```python
from build123d import *

# Parameters (mm, degrees)
MODEL_R             = 1.5
BOSS_EXTRUDE1_DEPTH = 3


with BuildPart() as part:
    # Model → Boss-Extrude1 (new body)
    with BuildSketch(Plane.XY):
        with BuildLine():
            Line((0.88624, 25.209039561), (0.88624, 11.208991882))
            ThreePointArc((0.88624, 11.208991882), (13.486238839, -1.391009279), (26.08624, 11.20898956))
            Line((26.08624, 11.20898956), (26.08624, 25.209041884))
            ThreePointArc((26.08624, 25.209041884), (13.486238839, 37.809039561), (0.88624, 25.209039561))
        make_face()
        with Locations((4.586289997, 18.209039557)):
            Circle(MODEL_R, mode=Mode.SUBTRACT)
        with Locations((22.586289997, 18.209039557)):
            Circle(MODEL_R, mode=Mode.SUBTRACT)
        Polygon((19.586238839, 6.708989561), (19.586238839, 29.708989561), (15.886238839, 29.708989561), (15.886238839, 31.708989561), (10.886238839, 31.708989561), (10.886238839, 29.708989561), (7.386238839, 29.708989561), (7.386238839, 6.708989561), align=None, mode=Mode.SUBTRACT)
    extrude(amount=BOSS_EXTRUDE1_DEPTH)


solid = part.part
```
Source: CAD feature listing. Evaluate the final solid. Frame: model axes, mm. A direction names the side the tool comes from. Round coordinates to 2 decimals unless told otherwise and drop trailing zeros. Write each loop counter-clockwise with the first axis right and the second up, starting at its lowest first coordinate (ties: lowest second). Pieces come first, ordered by that corner, then holes. Notation, with made-up numbers: M 34.25,32 L 75.25,32 A28 ccw 75.25,58 Z; hole C 12.25,16 d11. An arc over 180 degrees is marked long. Answer as a JSON object with one key per item and string values. Group by question number.
(1) Section query D-D on x = 7. Output: boundary loops of the cut face in (y, z).
(2) Mould query, pull axis Y, two halves, no side actions, for faces 1 (the flat face through (15.886, 31, 1)), 2 (the flat face through (22, 14, 3)), 3 (the cylindrical face through (13.209, -1.388, 1.479)). Classes: +Y half, -Y half, draft (parallel to the pull), parting line (faces both ways), or undercut.
(3) Section query B-B on z = 2.2. Output: boundary loops of the cut face in (x, y).
(4) Section query C-C on x = 10.5. Output: boundary loops of the cut face in (y, z), then the cut area to 3 significant figures.
(5) Reachability of faces 4 (the flat face through (7.386, 18, 1)), 5 (the flat face through (22, 14, 0)) from +Z, -Z, +X, -X, +Y, -Y: full face, straight path, thin tool, end or side. Return the list, or none.
(6) Ray query, line 1 (X direction, y = 18, z = 0.85); line 2 (X direction, y = 24.5, z = 1.8); line 3 (Y direction, x = 3.75, z = 1.6). Return the intervals inside material, ascending. Write a range as [from, to].
(7) Section query A-A on y = 13. Output: boundary loops of the cut face in (x, z), then the cut area to 3 significant figures.
(8) First-contact query: pin 1 (2.5 mm diameter, centred on x = 22.59, y = 18.21, fed in from +Z); pin 2 (0.9 mm diameter, centred on x = 18, z = 1, fed in from -Y); pin 3 (1 mm diameter, centred on y = 31, z = 2, fed in from -X); pin 4 (0.6 mm diameter, centred on y = 30.5, z = 1, fed in from +X). Flat tips, straight axial feed; report the tip coordinate or a pass-through.
Computed values:
{
 "1": {"outline": "M 0.41,0 L 36.01,0 L 36.01,3 L 0.41,3 Z"},
 "2": {"face 1": "undercut", "face 2": "draft", "face 3": "-Y half"},
 "3": {"outline": "M 0.89,11.21 A12.6 ccw 26.09,11.21 L 26.09,25.21 A12.6 ccw 0.89,25.21 Z; hole C 4.59,18.21 d3; hole M 7.39,6.71 L 19.59,6.71 L 19.59,29.71 L 15.89,29.71 L 15.89,31.71 L 10.89,31.71 L 10.89,29.71 L 7.39,29.71 Z; hole C 22.59,18.21 d3"},
 "4": {"outline": "M -1.03,0 L 6.71,0 L 6.71,3 L -1.03,3 Z; M 29.71,0 L 37.45,0 L 37.45,3 L 29.71,3 Z", "area": "46.4 mm^2"},
 "5": {"face 4": "+Z, -Z", "face 5": "-Z, +X, -X, +Y, -Y"},
 "6": {"line 1": "[0.89, 3.1], [6.07, 7.39], [19.59, 21.1], [24.07, 26.09]", "line 2": "[0.89, 7.39], [19.59, 26.09]", "line 3": "[3.21, 16.96], [19.45, 33.21]"},
 "7": {"outline": "M 0.89,0 L 7.39,0 L 7.39,3 L 0.89,3 Z; M 19.59,0 L 26.09,0 L 26.09,3 L 19.59,3 Z", "area": "39.0 mm^2"},
 "8": {"pin 1": "through", "pin 2": "y = -0.72", "pin 3": "x = 2.05", "pin 4": "x = 25.06"}
}
